Job drawing, mm, ordinate dimensions from the low corner. One solid piece. A direction names the side the tool comes from. Give positions to 0.01 mm unless a question says otherwise; leave off trailing zeros. Order: outer loops, then holes, each group sorted by start corner. A loop starts at its lowest first (then second) coordinate and runs counter-clockwise, first axis right, second up. Notation, with made-up numbers: M 5.5,5.5 L 22.5,5.5 A14 cw 22.5,11.5 Z; hole C 84.25,34.5 d8. An arc over 180 degrees is marked long. Put each result on its own line as item: value. Start each with the question number.
1) Cut at C-C (y = 23.25). Write the cut outline in (x, z).
2) Drill centre lines: line 1 (Z direction, x = 15.25, y = 2); line 2 (Z direction, x = 20.5, y = 2.5); line 3 (Y direction, x = 10.75, z = 29) (1 decimal). Where is each one in solid material? Low to high. Write a range as [from, to].
3) Tool access for the marked faces 1 and 2: list every direction of +Z, -Z, +X, -X, +Y, -Y with a clear straight run to the whole face (end or side of a thin tool).
4) Two-plate mould, pull along Z, no slides. Class the marked faces 3, 4 and 5: released by +Z, released by -Z, zero draft, split by the parting line, or undercut.
5) Cut at A-A (x = 12.7). Write the cut outline in (y, z) (1 decimal), and give its area (3 significant figures).
6) Cut at B-B (y = 3.5). Write the cut outline in (x, z), and give its area (3 significant figures).
7) Pin check, flat tip, straight feed: pin 1 (6 mm diameter, centred on x = 20.5, y = 15, fed in from +Z). Stop position of the tip, or through.
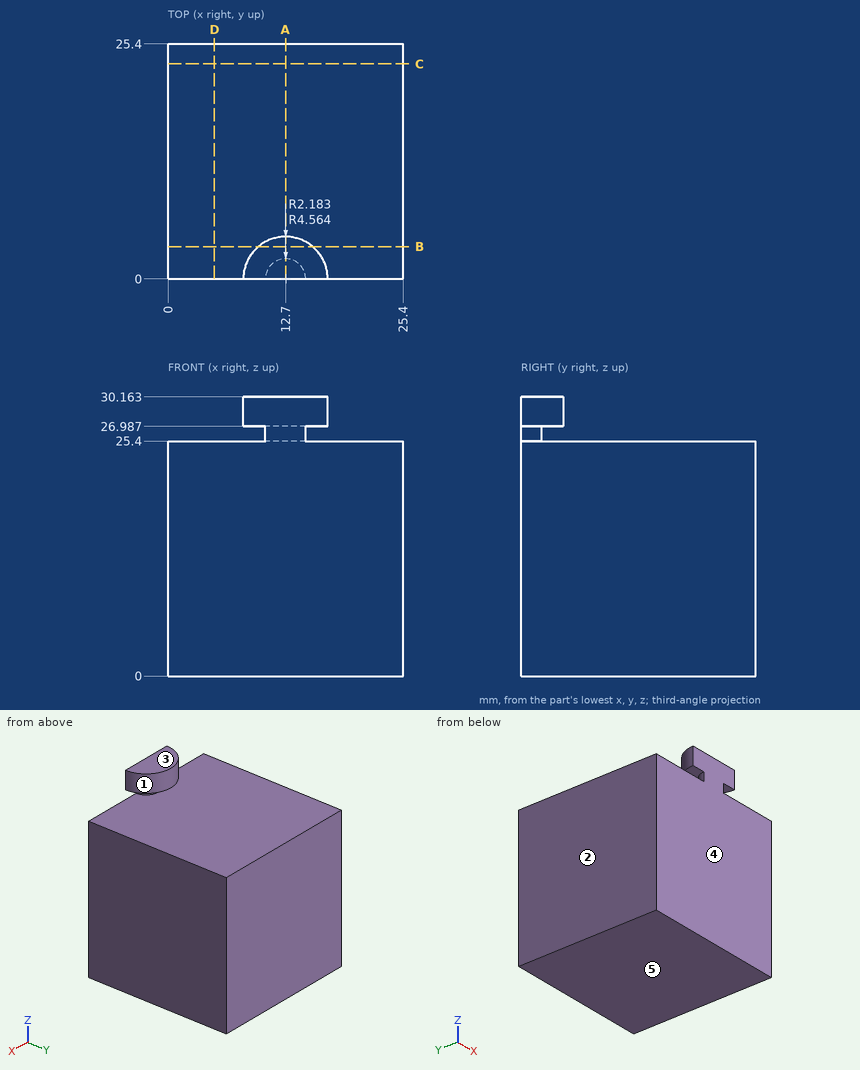
Solution:
1. outline: M 0,0 L 25.4,0 L 25.4,25.4 L 0,25.4 Z
2. line 1: [0, 25.4], [26.99, 30.16]
2. line 2: [0, 25.4]
2. line 3: [0, 4.1]
3. face 1: +Z, +Y
3. face 2: +Z, -Z, -X, +Y, -Y
4. face 3: released by +Z
4. face 4: zero draft
4. face 5: released by -Z
5. outline: M 0,0 L 25.4,0 L 25.4,25.4 L 2.2,25.4 L 2.2,27 L 4.6,27 L 4.6,30.2 L 0,30.2 Z
5. area: 663 mm²
6. outline: M 0,0 L 25.4,0 L 25.4,25.4 L 0,25.4 Z; M 9.77,26.99 L 15.63,26.99 L 15.63,30.16 L 9.77,30.16 Z
6. area: 664 mm²
7. pin 1: z = 25.4
